CAD build for the part. Positions are in the model's coordinates, mm. Give positions to 0.01 mm unless a question says otherwise; leave off trailing zeros. Order: outer loops, then holes, each group sorted by start corner. A loop starts at its lowest first (then second) coordinate and runs counter-clockwise, first axis right, second up.
Item 1: Wall check: L1, parallel to X at y = 17.25, z = 0; L2, parallel to X at y = 15.25, z = 2; L3, parallel to Z at x = -1, y = 2.25. Give the ranges that are in metal, low to high.
Item 2: Band-saw the part on D-D on z = 41. Give the cut face in (x, y).
Item 3: Flat gauge pins, fed straight in: P1, Ø6, axis at x = -8.5, y = 22, coming from the +Z side; P2, Ø8, axis at x = -29.5, y = 8.5, coming from the -Z side; P3, Ø4, axis at x = -41, z = 0, coming from the -Y side; P4, Ø2, axis at y = 9, z = 20.5, coming from the +X side. Where does each tip first touch, or does it go through?
Item 4: Band-saw the part on C-C on x = -21. Give the cut face in (y, z).
Item 5: Two-plate mould, pull along X, no slides. Class faces 1 (the flat face through (35, 28.7, 10)), 2 (the cylindrical face through (46.1, 14.1, -6.1)), 3 (the cylindrical face through (38.56, 14.55, -0.54)), 4 (the cylindrical face through (-26.513, 14.551, 28.666)): released by +X, released by -X, zero draft, split by the parting line, or undercut.
Item 6: Band-saw the part on B-B on z = 0. Give the cut face in (x, y), plus the area to 3 significant figures.
Item 7: Band-saw the part on A-A on x = 0. Give the cut face in (y, z).
```python
from build123d import *

# Parameters (mm, degrees)
SKETCH1_R           = 46.5
SKETCH1_R_2         = 36
BOSS_EXTRUDE1_DEPTH = 28.7
SKETCH2_R           = 2.5
CUT_EXTRUDE1_DEPTH  = 72.750888496


with BuildPart() as part:
    # Sketch1 → Boss-Extrude1 (new body)
    with BuildSketch(Plane(origin=(0, 0, 0), x_dir=(1, 0, 0), z_dir=(0, 1, 0))):
        with Locations(Location((0, 0, 0), (0, 0, 270))):
            Circle(SKETCH1_R)
        with Locations(Location((0, 0, 0), (0, 0, 270))):
            Circle(SKETCH1_R_2, mode=Mode.SUBTRACT)
    extrude(amount=BOSS_EXTRUDE1_DEPTH)

    # Sketch2 → Cut-Extrude1 (cut, through all)
    with BuildSketch(Plane(origin=(0, 28.7, 0), x_dir=(1, 0, 0), z_dir=(0, 1, 0))):
        with Locations(Location((0, 41, 0), (0, 0, 270))):
            Circle(SKETCH2_R)
        with Locations(Location((28.991378029, 28.991378029, 0), (0, 0, 270))):
            Circle(SKETCH2_R)
        with Locations(Location((41, 0, 0), (0, 0, 270))):
            Circle(SKETCH2_R)
        with Locations(Location((28.991378029, -28.991378029, 0), (0, 0, 270))):
            Circle(SKETCH2_R)
        with Locations(Location((0, -41, 0), (0, 0, 270))):
            Circle(SKETCH2_R)
        with Locations(Location((-28.991378029, -28.991378029, 0), (0, 0, 270))):
            Circle(SKETCH2_R)
        with Locations(Location((-41, 0, 0), (0, 0, 270))):
            Circle(SKETCH2_R)
        with Locations(Location((-28.991378029, 28.991378029, 0), (0, 0, 270))):
            Circle(SKETCH2_R)
    extrude(amount=-CUT_EXTRUDE1_DEPTH, mode=Mode.SUBTRACT)


solid = part.part
```
The answers:
1. L1: x = -46.5 to -43.5, -38.5 to -36, 36 to 38.5, 43.5 to 46.5
1. L2: x = -46.46 to -42.5, -39.5 to -35.94, 35.94 to 39.5, 42.5 to 46.46
1. L3: z = -46.49 to -43.29, -38.71 to -35.99, 35.99 to 38.71, 43.29 to 46.49
2. outline: (-21.94, 0) - (-2.5, 0) - (-2.5, 28.7) - (-21.94, 28.7) - close; (2.5, 0) - (21.94, 0) - (21.94, 28.7) - (2.5, 28.7) - close
3. P1: stops at z = 46.17
3. P2: stops at z = -38.88
3. P3: passes through
3. P4: stops at x = 42.21
4. outline: (0, -41.49) - (28.7, -41.49) - (28.7, -29.24) - (0, -29.24) - close; (0, 29.24) - (28.7, 29.24) - (28.7, 41.49) - (0, 41.49) - close
5. face 1: zero draft
5. face 2: split by the parting line
5. face 3: undercut
5. face 4: undercut
6. outline: (-46.5, 0) - (-43.5, 0) - (-43.5, 28.7) - (-46.5, 28.7) - close; (-38.5, 0) - (-36, 0) - (-36, 28.7) - (-38.5, 28.7) - close; (36, 0) - (38.5, 0) - (38.5, 28.7) - (36, 28.7) - close; (43.5, 0) - (46.5, 0) - (46.5, 28.7) - (43.5, 28.7) - close
6. area: 316 mm2
7. outline: (0, -46.5) - (28.7, -46.5) - (28.7, -43.5) - (0, -43.5) - close; (0, -38.5) - (28.7, -38.5) - (28.7, -36) - (0, -36) - close; (0, 36) - (28.7, 36) - (28.7, 38.5) - (0, 38.5) - close; (0, 43.5) - (28.7, 43.5) - (28.7, 46.5) - (0, 46.5) - close
